For this review, take the finished solid that the model builds, in its own axes (mm). Face numbers are marked on the shaded views. Coordinates: 2 decimals unless noted, no trailing zeros. Write each loop counter-clockwise with the first axis right and the second up, starting at its lowest first coordinate (ties: lowest second). Pieces come first, ordered by that corner, then holes.
```python
from build123d import *

# Parameters (mm, degrees)
F0_R     = 47.5
F0_R_2   = 27.5
F1_DEPTH = 30
F2_R     = 100
F2_R_2   = 47.5
F3_DEPTH = 3


with BuildPart() as f1:
    # F0 (on Right) → F1 (new body)
    with BuildSketch(Plane.YZ):
        Circle(F0_R)
        Circle(F0_R_2, mode=Mode.SUBTRACT)
    extrude(amount=F1_DEPTH)

    # F2 (on face) → F3 (join)
    with BuildSketch(Plane.YZ.offset(30)):
        Circle(F2_R)
        Circle(F2_R_2, mode=Mode.SUBTRACT)
    extrude(amount=-F3_DEPTH)

    # F4: F1 across face


with BuildPart() as f1_1:
    add(f1.part)
    add(f1.part.mirror(Plane(origin=(0, 0, 0), x_dir=(0, 1, 0), z_dir=(-1, 0, 0))))


solid = f1_1.part
```
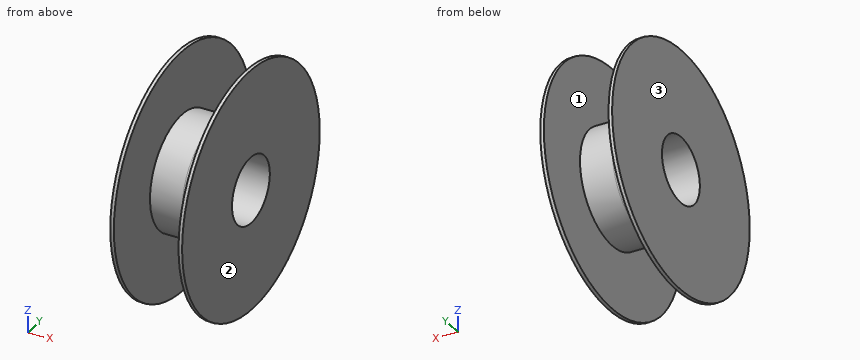
Q1. Add section C-C (x = 8.5). State the section outline as (y, z) points, then the cut area to 3 significant figures.
Ans:
outline: circle Ø95 at (0, 0); hole circle Ø55 at (0, 0)
area: 4,710 mm2
Q2. Clearance check with flat-ended pins moving along their axes: pin 1 Ø6 at (x, z) = (21, 33) entering from -Y; pin 2 Ø6 at (x, z) = (19, 19) entering from -Y. State where each tip first meets the part, or that it passes through.
Ans:
pin 1: stops at y = -36.83
pin 2: stops at y = -44.72
Q3. Add section A-A (z = 0). State the section outline as (x, y) points, then the cut area to 3 significant figures.
Ans:
outline: (-30, -100) - (-27, -100) - (-27, -47.5) - (27, -47.5) - (27, -100) - (30, -100) - (30, -27.5) - (-30, -27.5) - close; (-30, 27.5) - (30, 27.5) - (30, 100) - (27, 100) - (27, 47.5) - (-27, 47.5) - (-27, 100) - (-30, 100) - close
area: 3,030 mm2
Q4. For probe 1 along Z at (x, y) = (-7.25, 0); probe 2 along X at (y, z) = (-86, -5); probe 3 along Y at (x, z) = (-9.5, -15.5), list the stretches that pass through material, from the lowest coordinate up.
Ans:
probe 1: z = -47.5 to -27.5, 27.5 to 47.5
probe 2: x = -30 to -27, 27 to 30
probe 3: y = -44.9 to -22.72, 22.72 to 44.9
Q5. Add section D-D (y = 68). State the section outline as (x, z) points.
Ans:
outline: (-30, -73.32) - (-27, -73.32) - (-27, 73.32) - (-30, 73.32) - close; (27, -73.32) - (30, -73.32) - (30, 73.32) - (27, 73.32) - close
Q6. Draft analysis for pull direction X (two halves, no side actions). For the marked faces 1, 2 and 3, state which applies: +X half, -X half, draft (parallel to the pull), parting line (faces both ways), or undercut.
Ans:
face 1: undercut
face 2: +X half
face 3: -X half
